Geometry: final body of the model. Coordinates: model frame, mm. A direction names the side the tool comes from. Round coordinates to 2 decimals unless told otherwise and drop trailing zeros. Loops run counter-clockwise (first coordinate to the right, second up) from the corner with the lowest first, then second, coordinate; pieces in that order, holes last. Notation, with made-up numbers: (89.25, 61) - (142.25, 61) arc R22 ccw to (142.25, 96) - close; hole circle Ø2 at (-8, -14). An arc over 180 degrees is marked (long way). Answer as CSV lines item,"result".
from build123d import *

# Parameters (mm, degrees)
FILLET_1_R = 0.3


# Read off the part's stored shape, not the designer's step: Оболочка1
with BuildPart() as part:
    # Эскиз1 → Повернуть1 (revolve)
    with BuildSketch(Plane.XY, mode=Mode.PRIVATE) as revolve_1_sk:
        with BuildLine():
            Line((-12, -2.866025404), (-14, -2.866025404))
            Line((-14, -2.866025404), (-14, -3.866025404))
            Line((-14, -3.866025404), (0, -3.866025404))
            Line((0, -3.866025404), (0, 0))
            ThreePointArc((0, 0), (-5.942432162, -0.762343379), (-11.5, -3))
            ThreePointArc((-11.5, -3), (-11.741180955, -2.900099577), (-12, -2.866025404))
        make_face()
    revolve(revolve_1_sk.sketch.rotate(Axis((0, -3.866025404, 0), (0, 1, 0)), 270), axis=Axis((0, -3.866025404, 0), (0, 1, 0)))

    # Оболочка1 outline → Оболочка1 (revolve, cut)
    with BuildSketch(Plane.XY):
        with BuildLine():
            Line((0, -3.866025415), (10.999812609, -3.866025415))
            ThreePointArc((10.999812609, -3.866025415), (5.683528374, -1.728270752), (0, -1))
            Line((0, -1), (0, -3.866025415))
        make_face()
    revolve(axis=Axis((0, 0, 0), (0, 1, 0)), mode=Mode.SUBTRACT)

    # Скругление1
    fillet_1_edges = [part.edges().sort_by_distance(p)[0] for p in [
        (0, -3, 11.5),
    ]]
    fillet(fillet_1_edges, radius=FILLET_1_R)


solid = part.part
(1) Pin query (flat end, axial travel): P1, Ø1, axis at y = -3, z = 6.5, coming from the -X side; P2, Ø1.5, axis at x = 9.5, z = -9, coming from the +Y side; P3, Ø8.5, axis at x = -5.5, z = -4, coming from the +Y side. Return the tip coordinate at first contact, or that it passes through.
Findings below:
P1,"x = -12.65"
P2,"y = -2.87"
P3,"y = -0.14"
(2) Material intervals for line 1 along Z through (x, y) = (12.75, -2.95); line 2 along Y through (x, z) = (-5.5, -1.25); line 3 along Y through (x, z) = (-8.5, -6), sorted ascending.
Findings below:
line 1,"-5.78 to 5.78"
line 2,"-1.72 to -0.69"
line 3,"-3.54 to -2.42"
(3) Access query for faces 1 (the face through (9.3, -3.866, -6.2)), 2 (the face through (-10.4, -2.866, -6.3)). Directions: +Z, -Z, +X, -X, +Y, -Y. A direction counts if a zero-diameter tool reaches every point of the face in a straight line with its end or side. Return the directions, or none.
Findings below:
face 1,"+Z, -Z, +X, -X, -Y"
face 2,"+Y"
(4) Section A-A (y = -2.3). Output: boundary loops of the cut face in (x, z).
Findings below:
outline,"circle Ø20.3 at (0, 0); hole circle Ø15.09 at (0, 0)"
